Autodesk Inventor part; units mm, degrees
ref_plane "YZ Plane" through (0, 0, 0) normal (1, 0, 0) x (0, 1, 0)
ref_plane "XZ Plane" through (0, 0, 0) normal (0, 1, 0) x (-1, 0, 0)
ref_plane "XY Plane" through (0, 0, 0) normal (0, 0, 1) x (1, 0, 0)
sketch "Sketch1" plane through (0, 0, 0) normal (0, 1, 0) x (-1, 0, 0)
  line L0 (0, 279.3478) -> (-39.1304, 279.3478)
  line L1 (-39.1304, 279.3478) -> (-39.1304, -195.6522)
  line L2 (-39.1304, -195.6522) -> (0, -195.6522)
  line L3 (0, -195.6522) -> (0, 279.3478)
  line L4 (-39.1304, 279.3478) -> (-29.1304, 279.3478)
  line L5 (-29.1304, 254.3478) -> (-39.1304, 254.3478)
  line L6 (-39.1304, 254.3478) -> (-39.1304, 279.3478)
  line L7 (-39.1304, -195.6522) -> (-29.1304, -195.6522)
  line L8 (-29.1304, -170.6522) -> (-39.1304, -170.6522)
  line L9 (-39.1304, -170.6522) -> (-39.1304, -195.6522)
  point P0 (0, 0)
  point P1 (-39.1304, 254.3478)
  dimension "d0" = 475
  dimension "d4" = 25
  dimension "d5" = 25
extrude "Extrusion1" add sketch "Sketch1" along normal blind 160
sketch "Sketch2" plane through (0, 0, 279.3478) normal (0, 0, 1) x (1, 0, 0)
  line L0 (0, 160) -> (39.1304, 160)
  line L1 (0, 160) -> (39.1304, 160)
  line L2 (39.1304, 160) -> (39.1304, 0)
  line L3 (39.1304, 0) -> (0, 0)
  line L4 (0, 0) -> (0, 160)
  line L5 (39.1304, 160) -> (29.1304, 160)
  line L6 (29.1304, 160) -> (29.1304, 110)
  line L7 (29.1304, 110) -> (39.1304, 110)
  line L8 (39.1304, 110) -> (39.1304, 160)
  line L9 (39.1304, 0) -> (29.1304, 0)
  line L10 (29.1304, 0) -> (29.1304, 50)
  line L11 (29.1304, 50) -> (39.1304, 50)
  line L12 (39.1304, 50) -> (39.1304, 0)
  circle A0 centre (39.1304, 80) radius 18
  line L13 (31.1304, 75) -> (39.1304, 75)
  line L14 (39.1304, 75) -> (39.1304, 98)
  line L15 (39.1304, 98) -> (31.1304, 98)
  line L16 (31.1304, 98) -> (31.1304, 75)
  line L17 (31.1304, 75) -> (39.1304, 75)
  line L18 (39.1304, 75) -> (39.1304, 62)
  line L19 (39.1304, 62) -> (31.1304, 62)
  line L20 (31.1304, 62) -> (31.1304, 75)
  line L21 (39.1304, 0) -> (39.1304, 160)
  line L22 (0, 160) -> (19.1304, 160)
  line L23 (19.1304, 160) -> (19.1304, 0)
  line L24 (19.1304, 0) -> (0, 0)
  line L25 (0, 0) -> (0, 160)
  point P0 (0, 0)
  point P1 (34.1304, 110)
  point P2 (34.1304, 160)
  point P3 (39.1304, 50)
  point P4 (39.1304, 110)
  dimension "d6" = 10
  dimension "d7" = 50
  dimension "d8" = 50
  dimension "d9" = 8
  dimension "d10" = 36
  dimension "d11" = 80
  dimension "d12" = 80
  dimension "d15" = 20
extrude "Extrusion2" cut sketch "Sketch2" against normal up to surface (475 mm away) contours L0 L23 L3 L4 | L0 L2 L7 L6 | L10 L11 L2 L3 | L2 L13 L16 A0 | A0 L16 L15 | L2 A0 L20 L13 | L19 L20 A0
sketch "Sketch3" plane through (0, 160, 0) normal (0, 1, 0) x (1, 0, 0)
  line L0 (-18, 219) -> (160, 219)
  line L1 (160, 219) -> (160, 60.6522)
  line L2 (160, 60.6522) -> (-18, 60.6522)
  line L3 (-18, 60.6522) -> (-18, 219)
  line L4 (19.1304, -279.3478) -> (29.1304, -279.3478)
  point P0 (0, 0)
  dimension "d16" = 340
extrude "Extrusion3" cut sketch "Sketch3" against normal blind 200
sketch "Sketch4" plane through (39.1304, 98, 279.3478) normal (1, 0, 0) x (0, 0, -1)
  line L0 (340, 0) -> (340, 12)
  line L1 (340, 12) -> (0, 12)
  line L2 (0, 0) -> (0, 12)
  line L3 (0, 0) -> (340, 0)
  line L4 (340, -48) -> (340, -36)
  line L5 (340, -36) -> (0, -36)
  line L6 (0, -48) -> (0, -36)
  line L7 (0, -48) -> (340, -48)
  point P0 (279.3478, -98)
extrude "Extrusion4" add sketch "Sketch4" along normal blind 30
properties part number "MainRails" material "Aluminum 6061"
Work out the finished part from the listing and answer in its coordinate system (mm). A direction names the side the tool comes from. Round coordinates to 2 decimals unless told otherwise and drop trailing zeros. Loops run counter-clockwise (first coordinate to the right, second up) from the corner with the lowest first, then second, coordinate; pieces in that order, holes last. Notation, with made-up numbers: M 58.25,42 L 98.25,42 A35 ccw 98.25,74 Z; hole C 36,79 d2. An arc over 180 degrees is marked long. One line per question, with ' | ' between items.
Q1. Find section B-B, the plane z = -19.5. Give the vertices of the cut face in (x, y), then the cut area to 3 significant figures.
Conclusion:
outline: M 19.13,0 L 29.13,0 L 29.13,50 L 69.13,50 L 69.13,62 L 31.13,62 L 31.13,98 L 69.13,98 L 69.13,110 L 29.13,110 L 29.13,160 L 19.13,160 Z | area: 2,630 mm2
Q2. Consider line 1 along Y through (x, z) = (48, 176); line 2 along X through (y, z) = (129, 196.5); line 3 along X through (y, z) = (94, 195). Determine where each line is inside the solid, lowest interval first. Write a range as from..to.
Conclusion:
line 1: y = 50..62, 98..110 | line 2: x = 19.13..29.13 | line 3: x = 19.13..31.13
Q3. Find section C-C, the plane y = 20.5. Give the vertices of the cut face in (x, z).
Conclusion:
outline: M 19.13,-60.65 L 29.13,-60.65 L 29.13,279.35 L 19.13,279.35 Z
Q4. Find section D-D, the plane y = 84. Give the vertices of the cut face in (x, z), then the cut area to 3 significant figures.
Conclusion:
outline: M 19.13,-60.65 L 31.13,-60.65 L 31.13,279.35 L 19.13,279.35 Z | area: 4,080 mm2
Q5. A tool of negligible diameter and unlimited length cuts with its end or side. For faces 4 (the flat face through (31.13, 80, 112)), 5 (the flat face through (29.13, 25, 112)), 6 (the flat face through (29, 86, 279.348)), 7 (the flat face through (49, 110, 112)), from which of +Z, -Z, +X, -X, +Y, -Y can it reach the whole face along a straight path? Write none if from no direction.
Conclusion:
face 4: +Z, -Z, +X | face 5: +Z, -Z, +X, -Y | face 6: +Z, +X, -X, +Y, -Y | face 7: +Z, -Z, +X, +Y
Q6. Find section A-A, the plane x = 53.5. Give the vertices of the cut face in (y, z), then the cut area to 3 significant figures.
Conclusion:
outline: M 50,-60.65 L 62,-60.65 L 62,279.35 L 50,279.35 Z; M 98,-60.65 L 110,-60.65 L 110,279.35 L 98,279.35 Z | area: 8,160 mm2
Q7. The mould has two halves that part along Y. Classify faces 1 (the flat face through (24, 160, 112)), 2 (the flat face through (50, 62, 112)), 3 (the flat face through (29, 80, -60.652)): +Y half, -Y half, draft (parallel to the pull), parting line (faces both ways), or undercut.
Conclusion:
face 1: +Y half | face 2: undercut | face 3: draft
Q8. Each of these flat-tipped pins is pushed along its axis until it touches: pin 1 Ø15 at (y, z) = (23, 49.5) entering from +X; pin 2 Ø11.5 at (x, z) = (53.5, 48) entering from -Y; pin 3 Ø12 at (y, z) = (86.5, 139.5) entering from +X. Where does it stop, or does it pass through?
Conclusion:
pin 1: stops at x = 29.13 | pin 2: stops at y = 50 | pin 3: stops at x = 31.13
